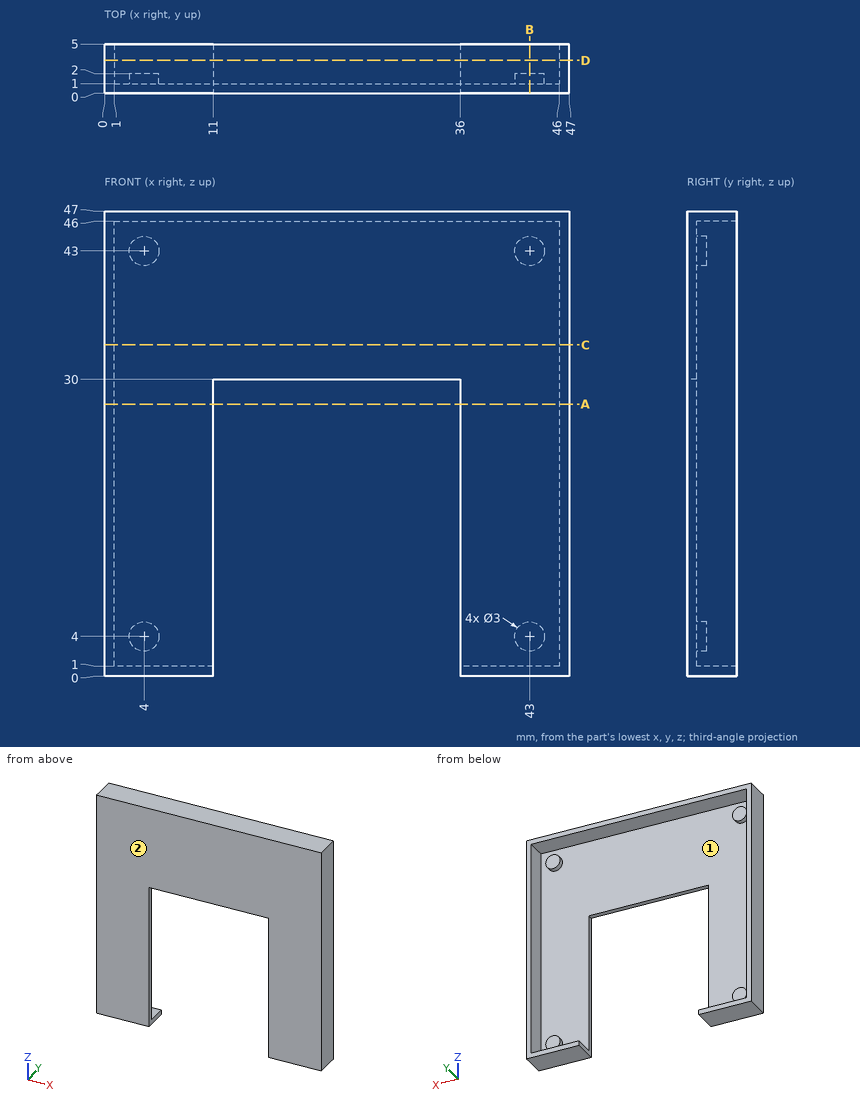
Could you check a few things on this drawing? It's one solid part, dimensions in mm from its lowest x, y, z. Coordinates: 2 decimals unless noted, no trailing zeros. Loops run counter-clockwise (first coordinate to the right, second up) from the corner with the lowest first, then second, coordinate; pieces in that order, holes last.
1. Imagine slicing it at C-C (z = 33.5). Please give me the cut outline in (x, y).
2. I need wall thicknesses on L1, parallel to Z at x = 37, y = 2.75; L2, parallel to X at y = 0.8, z = 20.5. Which ranges of each line are inside material? Lowest first, please.
3. Imagine slicing it at D-D (y = 3.35). Please give me the cut outline in (x, z).
4. For P1, Ø1.5, axis at x = 4.5, z = 4.5, coming from the +Y side; P2, Ø13.5, axis at x = 34, z = 24, coming from the +Y side; P3, Ø0.8, axis at x = 27.5, y = 0.5, coming from the -Z side, each with a flat end and sliding along its axis, tell me the tip position at first contact or that it passes through.
5. We'd pull the mould along X, two halves only. Please class the marked faces 1 and 2: released by +X, released by -X, zero draft, split by the parting line, or undercut.
6. Imagine slicing it at A-A (z = 27.5). Please give me the cut outline in (x, y), and give its area (3 significant figures).
7. Imagine slicing it at B-B (x = 43). Please give me the cut outline in (y, z), and give its area (3 significant figures).
Computed values:
1. outline: (0, 0) - (47, 0) - (47, 5) - (46, 5) - (46, 1) - (1, 1) - (1, 5) - (0, 5) - close
2. L1: z = 0 to 1, 46 to 47
2. L2: x = 0 to 11, 36 to 47
3. outline: (0, 0) - (11, 0) - (11, 1) - (1, 1) - (1, 46) - (46, 46) - (46, 1) - (36, 1) - (36, 0) - (47, 0) - (47, 47) - (0, 47) - close
4. P1: stops at y = 2
4. P2: stops at y = 1
4. P3: stops at z = 30
5. face 1: undercut
5. face 2: zero draft
6. outline: (0, 0) - (11, 0) - (11, 1) - (1, 1) - (1, 5) - (0, 5) - close; (36, 0) - (47, 0) - (47, 5) - (46, 5) - (46, 1) - (36, 1) - close
6. area: 30.0 mm2
7. outline: (0, 0) - (5, 0) - (5, 1) - (1, 1) - (1, 2.5) - (2, 2.5) - (2, 5.5) - (1, 5.5) - (1, 41.5) - (2, 41.5) - (2, 44.5) - (1, 44.5) - (1, 46) - (5, 46) - (5, 47) - (0, 47) - close
7. area: 61.0 mm2
